Could you check a few things on this model? Use its own coordinates, in mm. A direction names the side the tool comes from. Give positions to 0.01 mm unless a question says otherwise; leave off trailing zeros. Loops run counter-clockwise (first coordinate to the right, second up) from the corner with the lowest first, then second, coordinate; pieces in that order, holes last. Notation, with made-up numbers: (59.25, -35.75) - (112.25, -35.75) arc R19 cw to (112.25, -29.75) - close; hole circle Ø3 at (-30, 12). An arc over 180 degrees is marked (long way). Write each question's results on one line, items separated by ' | '. Start each with the question number.
```python
from build123d import *

# Parameters (mm, degrees)
EXTRUDE_1_DEPTH            = 18
EXTRUDE_1_DEPTH_BACK       = 18
SHELL_START                = -16
SHELL_1_DEPTH              = 32
EXTRUDE_START              = 5.2
SKETCH_3_R                 = 1.5
EXTRUDE_4_DEPTH            = 2
SKETCH_4_W                 = 3.4
SKETCH_4_H                 = 6
CUT_EXTRUDE_1_DEPTH        = 10
PATTERN_LINEAR_1_COUNT     = 3
PATTERN_LINEAR_1_PITCH     = 6.5
PATTERN_LINEAR_1_COL_COUNT = 3
PATTERN_LINEAR_1_COL_PITCH = 6.5
FILLET_1_R                 = 1


# Read off the part's stored shape, not the designer's step: 抽壳1
with BuildPart() as part:
    # 草图1 → 凸台-拉伸1 (new, two sides: drawn at the far end of the back side and taken through both)
    with BuildSketch(Plane.XY.offset(-EXTRUDE_1_DEPTH_BACK)):
        with BuildLine():
            Line((151.788918014, 43.508002681), (159.327869649, 39.07926315))
            ThreePointArc((159.327869649, 39.07926315), (161.564024285, 38.110077711), (163.968213283, 37.710599005))
            Line((163.968213283, 37.710599005), (192.119395463, 36.513624191))
            Line((192.119395463, 36.513624191), (192.119395463, 24.680778737))
            Line((192.119395463, 24.680778737), (190.423481116, 18.459832962))
            ThreePointArc((190.423481116, 18.459832962), (186.255085289, 12.72488885), (179.332402452, 11.194669891))
            ThreePointArc((179.332402452, 11.194669891), (174.394698317, 13.051819811), (170.680138106, 16.797746984))
            Line((170.680138106, 16.797746984), (151.788918014, 43.508002681))
        make_face()
    extrude(amount=EXTRUDE_1_DEPTH + EXTRUDE_1_DEPTH_BACK)

    # 抽壳1 outline → 抽壳1 (cut)
    with BuildSketch(Plane.XY.offset(SHELL_START)):
        with BuildLine():
            Line((190.119395463, 24.94850719), (190.119395463, 36.598663235))
            Line((190.119395463, 36.598663235), (163.968213283, 37.710599005))
            ThreePointArc((163.968213283, 37.710599005), (161.564024285, 38.110077711), (159.327869649, 39.07926315))
            Line((159.327869649, 39.07926315), (155.979837332, 41.046056915))
            Line((155.979837332, 41.046056915), (172.342749657, 17.910570164))
            ThreePointArc((172.342749657, 17.910570164), (175.462047648, 14.743395572), (179.621034868, 13.173733136))
            ThreePointArc((179.621034868, 13.173733136), (185.159181138, 14.397908304), (188.493897799, 18.985863593))
            Line((188.493897799, 18.985863593), (190.119395463, 24.94850719))
        make_face()
    extrude(amount=SHELL_1_DEPTH, mode=Mode.SUBTRACT)

    # 草图3 → 凸台-拉伸4 (add)
    with BuildSketch(Plane.XY.offset(EXTRUDE_START)):
        with BuildLine():
            Line((195.035842319, 39.575477762), (190.226405911, 36.594113202))
            Line((190.226405911, 36.594113202), (192.119395463, 36.513624191))
            Line((192.119395463, 36.513624191), (192.119395463, 24.680778737))
            Line((192.119395463, 24.680778737), (191.271438289, 21.570305849))
            Line((191.271438289, 21.570305849), (197.536771011, 20.886144131))
            ThreePointArc((197.536771011, 20.886144131), (199.439234753, 21.918899338), (200.054211557, 23.99441256))
            Line((200.054211557, 23.99441256), (199.013675467, 38.561520293))
            ThreePointArc((199.013675467, 38.561520293), (197.234756361, 39.892335247), (195.035842319, 39.575477762))
        make_face()
        with Locations((197.241357069, 23.698998619)):
            Circle(SKETCH_3_R, mode=Mode.SUBTRACT)
        with Locations((196.517780159, 36.376109938)):
            Circle(SKETCH_3_R, mode=Mode.SUBTRACT)
    extrude_4 = extrude(amount=EXTRUDE_4_DEPTH)

    # 镜向1: 凸台-拉伸4 across plane
    add(extrude_4.mirror(Plane.XY))

    # 草图4 → 切除-拉伸1 (cut)
    with BuildSketch(Plane(origin=(121.688944553, 86.066290803, 0), x_dir=(0, 0, 1), z_dir=(-0.8164358107895011, -0.577436201549998, 0))):
        with Locations((0, -55.12692481)):
            Rectangle(SKETCH_4_W, SKETCH_4_H)
    cut_extrude_1 = extrude(amount=-CUT_EXTRUDE_1_DEPTH, mode=Mode.SUBTRACT)

    # 阵列(线性)1: 切除-拉伸1 ×3
    with Locations(*[(0, 0, -i * PATTERN_LINEAR_1_PITCH) for i in range(1, PATTERN_LINEAR_1_COUNT)]):
        add(cut_extrude_1, mode=Mode.SUBTRACT)

    # 阵列(线性)1 col: 切除-拉伸1 ×3
    with Locations(*[(0, 0, i * PATTERN_LINEAR_1_COL_PITCH) for i in range(1, PATTERN_LINEAR_1_COL_COUNT)]):
        add(cut_extrude_1, mode=Mode.SUBTRACT)

    # 圆角1
    fillet_1_edges = [part.edges().sort_by_distance(p)[0] for p in [
        (156.069971034, 39.186824018, -1.7),
        (156.069971034, 39.186824018, 1.7),
        (156.069971034, 39.186824018, 4.8),
        (156.069971034, 39.186824018, 8.2),
        (156.069971034, 39.186824018, 11.3),
        (156.069971034, 39.186824018, 14.7),
        (156.069971034, 39.186824018, -8.2),
        (156.069971034, 39.186824018, -4.8),
        (156.069971034, 39.186824018, -14.7),
        (156.069971034, 39.186824018, -11.3),
    ]]
    fillet(fillet_1_edges, radius=FILLET_1_R)


solid = part.part
```
Q1. Which directions (+Z, -Z, +X, -X, +Y, -Y) give clear straight access to the entire face, cutting with the end or side of a thin tool? Please do faces 1 (the face through (192.119, 31, -13)), 2 (the face through (192.665, 38.106, 6.186)), 3 (the face through (161.53, 38.12, -17.01)), 4 (the face through (155.908, 39.44, 14.415)).
Q2. I'm going to push flat-ended pins straight in: pin 1 Ø6 at (y, z) = (21, 3) entering from -X; pin 2 Ø8 at (y, z) = (34, -6) entering from +X; pin 3 Ø8 at (x, y) = (197.5, 29) entering from +Z. Where does each tip first touch, or does it pass through?
Q3. If we mould it in two halves opening along X, with no side actions, what happens to faces 5 (the face through (154.7, 41.8, 16.7)), 6 (the face through (155.908, 39.44, -11.585)), 7 (the face through (185.091, 14.354, -0.224))? For each: +X half, -X half, draft (parallel to the pull), parting line (faces both ways), or undercut.
Q4. I want a section at A-A, the plane y = 23. List the corners of the cut face in (x, z) for me.
Q5. I want a section at D-D, the plane y = 14. List the corners of the cut face in (x, z) for me (3 decimals), then the cut area to 3 significant figures.
Q6. I need wall thicknesses on L1, parallel to Z at x = 176.5, y = 28.5; L2, parallel to Z at x = 198, y = 27; L3, parallel to X at y = 22.5, z = 4. Which ranges of each line are inside material? Lowest first, please. Write a range as from..to.
Q7. I want a section at B-B, the plane z = -9. List the corners of the cut face in (x, y) for me, then the cut area to 3 significant figures.
Q8. I want a section at C-C, the plane x = 194. List the corners of the cut face in (y, z) for me.
Conclusion:
1) face 1: -Z, +X, +Y, -Y | face 2: +Z, -Z, +Y | face 3: +Z, -Z, +X, +Y | face 4: -X, +Y
2) pin 1: x = 165.59 | pin 2: x = 199.63 | pin 3: z = 7.2
3) face 5: +X half | face 6: -X half | face 7: undercut
4) outline: (166.29, -18) - (191.66, -18) - (191.66, -7.2) - (195.91, -7.2) - (195.91, -5.2) - (191.66, -5.2) - (191.66, 5.2) - (195.91, 5.2) - (195.91, 7.2) - (191.66, 7.2) - (191.66, 18) - (166.29, 18) - close; (198.57, -7.2) - (199.98, -7.2) - (199.98, -5.2) - (198.57, -5.2) - close; (198.57, 5.2) - (199.98, 5.2) - (199.98, 7.2) - (198.57, 7.2) - close; hole (168.74, -16) - (189.59, -16) - (189.59, 16) - (168.74, 16) - close
5) outline: (173.119, -18) - (187.828, -18) - (187.828, 18) - (173.119, 18) - close; hole (176.815, -16) - (184.481, -16) - (184.481, 16) - (176.815, 16) - close | area: 284 mm^2
6) L1: -18..-16, 16..18 | L2: -7.2..-5.2, 5.2..7.2 | L3: 166.65..169.1, 189.45..191.52
7) outline: (151.79, 43.51) - (170.68, 16.8) arc R12.37 ccw to (179.33, 11.19) arc R10 ccw to (190.42, 18.46) - (192.12, 24.68) - (192.12, 36.51) - (190.12, 36.6) - (190.12, 24.95) - (188.49, 18.99) arc R8 cw to (179.62, 13.17) arc R10.37 cw to (172.34, 17.91) - (155.98, 41.05) - close | area: 143 mm^2
8) outline: (21.27, -7.2) - (38.93, -7.2) - (38.93, -5.2) - (21.27, -5.2) - close; (21.27, 5.2) - (38.93, 5.2) - (38.93, 7.2) - (21.27, 7.2) - close
